Read the model definition and answer for the solid it produces. Units are mm, in the model's axes. Round coordinates to 2 decimals unless told otherwise and drop trailing zeros. Order: outer loops, then holes, each group sorted by start corner. A loop starts at its lowest first (then second) coordinate and runs counter-clockwise, first axis right, second up. Notation, with made-up numbers: (61.5, 76.5) -> (76.5, 76.5) arc R23 cw to (76.5, 96.5) -> close; hole circle Ø2 at (71, 5.5). An arc over 180 degrees is marked (long way). Use a Markdown table: item, result. Add a question column.
1. Section D-D, the plane y = -70.5 is taken. Give the vertices of the cut face in (x, z), then the cut area to 3 significant figures.
2. Section B-B, the plane y = -86.25 is taken. Give the vertices of the cut face in (x, z).
3. Section C-C, the plane z = 2.45 is taken. Give the number of separate pieces and of enclosed holes in the cut face, then the cut area to 3 significant figures.
4. Section A-A, the plane x = -35 is taken. Give the vertices of the cut face in (y, z), then the cut area to 3 significant figures.
5. Consider L1, parallel to Y at x = 7.5, z = 2.4; L2, parallel to Y at x = 5, z = 1.95; L3, parallel to X at y = -41, z = 2.9. Determine where each line is inside the solid, lowest interval first. Write a range as [from, to].
6. Given pin 1 (2.5 mm diameter, centred on x = -35, y = -86.25, fed in from +Z); pin 2 (0.9 mm diameter, centred on x = -16, z = 1.5, fed in from +Y) (3 decimals), each flat-ended and moving along its own axis, determine where each tip first touches the part or whether it passes through.
```python
from build123d import *

# Parameters (mm, degrees)
EXTRUDE_1_DEPTH     = 3
SKETCH_2_R          = 1.6
SKETCH_2_W          = 1.5
SKETCH_2_H          = 17
CUT_EXTRUDE_1_DEPTH = 118.192149908


with BuildPart() as part:
    # 草图1 → 凸台-拉伸1 (new body)
    with BuildSketch(Plane.XY):
        Polygon((0, 0), (20, 0), (75, -75), (75, -90), (-50, -90), (-50, -75), align=None)
    extrude(amount=EXTRUDE_1_DEPTH)

    # 草图2 → 切除-拉伸1 (cut, through all)
    with BuildSketch(Plane.XY.offset(3)):
        with Locations((5, -5)):
            Circle(SKETCH_2_R)
        with Locations(Location((15, -5, 0), (0, 0, 180))):
            Circle(SKETCH_2_R)
        with Locations((15, -15)):
            Circle(SKETCH_2_R)
        with Locations(Location((5, -15, 0), (0, 0, 180))):
            Circle(SKETCH_2_R)
        with Locations((-45, -86.25)):
            Circle(SKETCH_2_R)
        with Locations(Location((-45, -78.75, 0), (0, 0, 180))):
            Circle(SKETCH_2_R)
        with Locations(Location((-35, -86.25, 0), (0, 0, 180))):
            Circle(SKETCH_2_R)
        with Locations((-35, -78.75)):
            Circle(SKETCH_2_R)
        with Locations(Location((60, -78.75, 0), (0, 0, 180))):
            Circle(SKETCH_2_R)
        with Locations((60, -86.25)):
            Circle(SKETCH_2_R)
        with Locations((70, -78.75)):
            Circle(SKETCH_2_R)
        with Locations(Location((70, -86.25, 0), (0, 0, 180))):
            Circle(SKETCH_2_R)
        with Locations((7.5, -86.25)):
            Circle(SKETCH_2_R)
        with Locations(Location((17.5, -86.25, 0), (0, 0, 180))):
            Circle(SKETCH_2_R)
        with Locations((17.5, -78.75)):
            Circle(SKETCH_2_R)
        with Locations(Location((7.5, -78.75, 0), (0, 0, 180))):
            Circle(SKETCH_2_R)
        with Locations((5, -45)):
            Circle(SKETCH_2_R)
        with Locations(Location((15, -45, 0), (0, 0, 180))):
            Circle(SKETCH_2_R)
        with Locations((15, -55)):
            Circle(SKETCH_2_R)
        with Locations(Location((5, -55, 0), (0, 0, 180))):
            Circle(SKETCH_2_R)
        Polygon((-2, -30.041634566), (-2, -72.5), (-30.305576956, -72.5), align=None)
        Polygon((22, -72.5), (50.305576956, -72.5), (22, -30.041634566), align=None)
        with Locations((74.25, -81.5)):
            Rectangle(SKETCH_2_W, SKETCH_2_H)
        with Locations((-49.25, -81.5)):
            Rectangle(SKETCH_2_W, SKETCH_2_H)
    extrude(amount=-CUT_EXTRUDE_1_DEPTH, mode=Mode.SUBTRACT)


solid = part.part
```
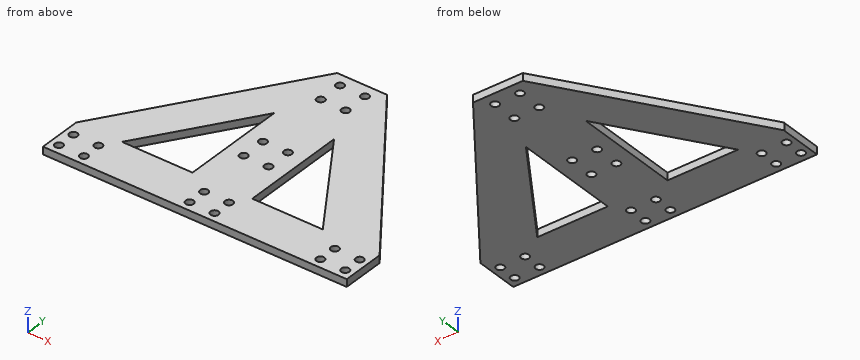
Verdict:
| question | item | result |
|---|---|---|
| 1 | outline | (-47, 0) -> (-28.97, 0) -> (-28.97, 3) -> (-47, 3) -> close; (-2, 0) -> (22, 0) -> (22, 3) -> (-2, 3) -> close; (48.97, 0) -> (71.7, 0) -> (71.7, 3) -> (48.97, 3) -> close |
| 1 | area | 194 mm2 |
| 2 | outline | (-48.5, 0) -> (-46.6, 0) -> (-46.6, 3) -> (-48.5, 3) -> close; (-43.4, 0) -> (-36.6, 0) -> (-36.6, 3) -> (-43.4, 3) -> close; (-33.4, 0) -> (5.9, 0) -> (5.9, 3) -> (-33.4, 3) -> close; (9.1, 0) -> (15.9, 0) -> (15.9, 3) -> (9.1, 3) -> close; (19.1, 0) -> (58.4, 0) -> (58.4, 3) -> (19.1, 3) -> close; (61.6, 0) -> (68.4, 0) -> (68.4, 3) -> (61.6, 3) -> close; (71.6, 0) -> (73.5, 0) -> (73.5, 3) -> (71.6, 3) -> close |
| 3 | separate pieces | 1 |
| 3 | enclosed holes | 22 |
| 3 | area | 5,900 mm2 |
| 4 | outline | (-90, 0) -> (-87.85, 0) -> (-87.85, 3) -> (-90, 3) -> close; (-84.65, 0) -> (-80.35, 0) -> (-80.35, 3) -> (-84.65, 3) -> close; (-77.15, 0) -> (-52.5, 0) -> (-52.5, 3) -> (-77.15, 3) -> close |
| 4 | area | 93.3 mm2 |
| 5 | L1 | y = [-90, -87.85], [-84.65, -80.35], [-77.15, 0] |
| 5 | L2 | y = [-90, -56.6], [-53.4, -46.6], [-43.4, -16.6], [-13.4, -6.6], [-3.4, 0] |
| 5 | L3 | x = [-27.33, -9.31], [-2, 22], [29.31, 50.07] |
| 6 | pin 1 | passes through |
| 6 | pin 2 | stops at y = -23.325 |
